from build123d import *

# Parameters (mm, degrees)
EXTRUDE_1_DEPTH     = 15
EXTRUDE_2_DEPTH     = 6.51
CUT_EXTRUDE_1_DEPTH = 4.65
CHAMFER_1_SIZE      = 0.1
FILLET_1_R          = 0.25
CUT_EXTRUDE_2_DEPTH = 0.2
SKETCH_5_R          = 2.5
EXTRUDE_3_DEPTH     = 8
FILLET_2_R          = 0.25
SKETCH_6_R          = 1.5
EXTRUDE_4_DEPTH     = 8


with BuildPart() as part:
    # Эскиз1 → Бобышка-Вытянуть1 (new body)
    with BuildSketch(Plane.XY):
        with BuildLine():
            Line((-2.925, 3.25), (2.925, 3.25))
            ThreePointArc((2.925, 3.25), (6.175, 0), (2.925, -3.25))
            Line((2.925, -3.25), (-2.925, -3.25))
            ThreePointArc((-2.925, -3.25), (-6.175, 0), (-2.925, 3.25))
        make_face()
    extrude(amount=EXTRUDE_1_DEPTH)

    # Эскиз2 → Бобышка-Вытянуть2 (add)
    with BuildSketch(Plane(origin=(0, 0, 0), x_dir=(-1, 0, 0), z_dir=(0, 0, -1))):
        with BuildLine():
            Line((-2.925, 1.2), (2.925, 1.2))
            ThreePointArc((2.925, 1.2), (4.125, 0), (2.925, -1.2))
            Line((2.925, -1.2), (-2.925, -1.2))
            ThreePointArc((-2.925, -1.2), (-4.125, 0), (-2.925, 1.2))
        make_face()
    extrude(amount=EXTRUDE_2_DEPTH)

    # Эскиз3 → Вырез-Вытянуть1 (cut)
    with BuildSketch(Plane(origin=(0, 0, -6.51), x_dir=(-1, 0, 0), z_dir=(0, 0, -1))):
        with BuildLine():
            Line((-2.944601233, -0.65), (2.944601233, -0.65))
            ThreePointArc((2.944601233, -0.65), (3.214554933, -0.579192028), (3.415, -0.385))
            Line((3.415, -0.385), (3.415, 0.385))
            ThreePointArc((3.415, 0.385), (3.214554933, 0.579192028), (2.944601233, 0.65))
            Line((2.944601233, 0.65), (-2.944601233, 0.65))
            ThreePointArc((-2.944601233, 0.65), (-3.214554933, 0.579192028), (-3.415, 0.385))
            Line((-3.415, 0.385), (-3.415, -0.385))
            ThreePointArc((-3.415, -0.385), (-3.214554933, -0.579192028), (-2.944601233, -0.65))
        make_face()
    extrude(amount=-CUT_EXTRUDE_1_DEPTH, mode=Mode.SUBTRACT)

    # Фаска1
    chamfer_1_edges = [part.edges().sort_by_distance(p)[0] for p in [
        (3.214554933, -0.579192028, -6.51),
        (-3.214554933, -0.579192028, -6.51),
        (0, -0.65, -6.51),
    ]]
    chamfer(chamfer_1_edges, length=CHAMFER_1_SIZE)
    chamfer_1_2_edges = [part.edges().sort_by_distance(p)[0] for p in [
        (3.214554933, 0.579192028, -6.51),
        (0, 0.65, -6.51),
        (-3.214554933, 0.579192028, -6.51),
    ]]
    chamfer(chamfer_1_2_edges, length=CHAMFER_1_SIZE)
    chamfer_1_3_edges = [part.edges().sort_by_distance(p)[0] for p in [
        (-3.415, 0, -6.51),
    ]]
    chamfer(chamfer_1_3_edges, length=CHAMFER_1_SIZE - 0.0001)  # a hair under: the kernel refuses the full size
    chamfer_1_4_edges = [part.edges().sort_by_distance(p)[0] for p in [
        (3.415, 0, -6.51),
    ]]
    chamfer(chamfer_1_4_edges, length=CHAMFER_1_SIZE)

    # Скругление1
    fillet_1_edges = [part.edges().sort_by_distance(p)[0] for p in [
        (4.125, 0, -6.51),
        (0, -1.2, -6.51),
        (-4.125, 0, -6.51),
        (0, 1.2, -6.51),
    ]]
    fillet(fillet_1_edges, radius=FILLET_1_R)

    # Эскиз4 → Вырез-Вытянуть2 (cut)
    with BuildSketch(Plane(origin=(0, 3.25, 0), x_dir=(1, 0, 0), z_dir=(0, 1, 0))):
        with BuildLine():
            Line((-2.5, -2.5), (2.5, -2.5))
            ThreePointArc((2.5, -2.5), (2.679605122, -2.574394878), (2.754, -2.754))
            Line((2.754, -2.754), (2.754, -12.246))
            ThreePointArc((2.754, -12.246), (2.679605122, -12.425605122), (2.5, -12.5))
            Line((2.5, -12.5), (-2.5, -12.5))
            ThreePointArc((-2.5, -12.5), (-2.679605122, -12.425605122), (-2.754, -12.246))
            Line((-2.754, -12.246), (-2.754, -2.754))
            ThreePointArc((-2.754, -2.754), (-2.679605122, -2.574394878), (-2.5, -2.5))
        make_face()
        with BuildLine():
            Line((0, -2.878550244), (-0.716956191, -3.598432054))
            Line((-0.716956191, -3.598432054), (-0.127, -3.598432054))
            Line((-0.127, -3.598432054), (-0.127, -9.006251958))
            ThreePointArc((-0.127, -9.006251958), (-0.156162493, -9.052213445), (-0.21016765, -9.045405185))
            Line((-0.21016765, -9.045405185), (-1.120514747, -8.292828766))
            ThreePointArc((-1.120514747, -8.292828766), (-1.324422308, -8.030092949), (-1.397, -7.705530349))
            Line((-1.397, -7.705530349), (-1.397, -6.445060748))
            ThreePointArc((-1.397, -6.445060748), (-1.524, -5.445191863), (-1.651, -6.445060748))
            Line((-1.651, -6.445060748), (-1.651, -7.68561956))
            ThreePointArc((-1.651, -7.68561956), (-1.550201428, -8.136384053), (-1.267007097, -8.501281232))
            Line((-1.267007097, -8.501281232), (-0.219161751, -9.367526318))
            ThreePointArc((-0.219161751, -9.367526318), (-0.151192564, -9.455104923), (-0.127, -9.563292457))
            Line((-0.127, -9.563292457), (-0.127, -10.838615444))
            ThreePointArc((-0.127, -10.838615444), (0, -12.095785839), (0.127, -10.838615444))
            Line((0.127, -10.838615444), (0.127, -8.47461517))
            ThreePointArc((0.127, -8.47461517), (0.139930568, -8.394605616), (0.177405738, -8.322742274))
            Line((0.177405738, -8.322742274), (1.053118903, -7.148798926))
            ThreePointArc((1.053118903, -7.148798926), (1.165544414, -6.933208901), (1.204336117, -6.693180239))
            Line((1.204336117, -6.693180239), (1.204336117, -5.889691863))
            Line((1.204336117, -5.889691863), (1.524, -5.889691863))
            Line((1.524, -5.889691863), (1.524, -5.000691863))
            Line((1.524, -5.000691863), (0.635, -5.000691863))
            Line((0.635, -5.000691863), (0.635, -5.889691863))
            Line((0.635, -5.889691863), (0.954663883, -5.889691863))
            Line((0.954663883, -5.889691863), (0.954663883, -6.609767291))
            ThreePointArc((0.954663883, -6.609767291), (0.915872181, -6.849795953), (0.80344667, -7.065385978))
            Line((0.80344667, -7.065385978), (0.218518852, -7.849515015))
            ThreePointArc((0.218518852, -7.849515015), (0.161798089, -7.867354322), (0.127, -7.819140435))
            Line((0.127, -7.819140435), (0.127, -3.598432054))
            Line((0.127, -3.598432054), (0.716956191, -3.598432054))
            Line((0.716956191, -3.598432054), (0, -2.878550244))
        make_face(mode=Mode.SUBTRACT)
    extrude(amount=-CUT_EXTRUDE_2_DEPTH, mode=Mode.SUBTRACT)

    # Эскиз5 → Бобышка-Вытянуть3 (add)
    with BuildSketch(Plane.XY.offset(15)):
        Circle(SKETCH_5_R)
    extrude(amount=EXTRUDE_3_DEPTH)

    # Скругление2
    fillet_2_edges = [part.edges().sort_by_distance(p)[0] for p in [
        (6.175, 0, 15),
        (0, 3.25, 15),
        (-2.5, 0, 23),
        (-6.175, 0, 15),
        (0, 3.25, 0),
        (6.175, 0, 0),
        (0, -3.25, 0),
        (-6.175, 0, 0),
        (0, -3.25, 15),
    ]]
    fillet(fillet_2_edges, radius=FILLET_2_R)

    # Эскиз6 → Бобышка-Вытянуть4 (add)
    with BuildSketch(Plane.XY.offset(23)):
        Circle(SKETCH_6_R)
    extrude(amount=EXTRUDE_4_DEPTH)


solid = part.part
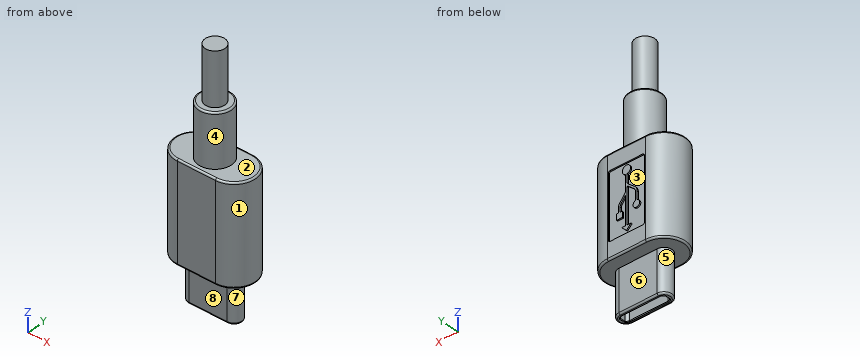
Read the model definition and answer for the solid it produces. Units are mm, in the model's axes. Face numbers are marked on the shaded views. A direction names the side the tool comes from. Round coordinates to 2 decimals unless told otherwise and drop trailing zeros. Loops run counter-clockwise (first coordinate to the right, second up) from the corner with the lowest first, then second, coordinate; pieces in that order, holes last.
Q1. Which of the six approach directions +Z, -Z, +X, -X, +Y, -Y give full straight-line access (tool end or side, diameter ignored) to the marked faces 4, 5, 6, 7 and 8?
Q2. Consider probe 1 along X at (y, z) = (-1.25, 4) (3 decimals); probe 2 along Z at (x, y) = (4.75, -0.5); probe 3 along Y at (x, z) = (-2.5, 7). Determine where each line is inside the solid, lowest interval first.
Q3. Each of these flat-tipped pins is pushed along its axis until it touches: pin 1 (3 mm diameter, centred on x = -3.5, y = 1.5, fed in from +Z); pin 2 (3.5 mm diameter, centred on x = 1.5, z = -3, fed in from +Y); pin 3 (1.4 mm diameter, centred on x = 0.5, y = 0, fed in from -Z). Where does it stop, or does it pass through?
Q4. Section B-B on z = 14 is taken. Write down the section's boundary in (x, y) (3 decimals).
Q5. Determine the mould class of the marked faces 1, 2 and 3 for opening direction Z: released by +Z, released by -Z, zero draft, split by the parting line, or undercut.
Output:
1. face 4: +Z
1. face 5: -Z, -X
1. face 6: -Z, +X, -X, +Y
1. face 7: -Z, +X
1. face 8: -Z, +X, -X, -Y
2. probe 1: x = -5.925 to 5.925
2. probe 2: z = 0 to 15
2. probe 3: y = -3.25 to 3.05
3. pin 1: stops at z = 22.99
3. pin 2: stops at y = 1.2
3. pin 3: stops at z = -6.46
4. outline: (-2.925, -3.25) - (2.925, -3.25) arc R3.25 ccw to (2.925, 3.25) - (-2.925, 3.25) arc R3.25 ccw to start
5. face 1: zero draft
5. face 2: released by +Z
5. face 3: undercut
